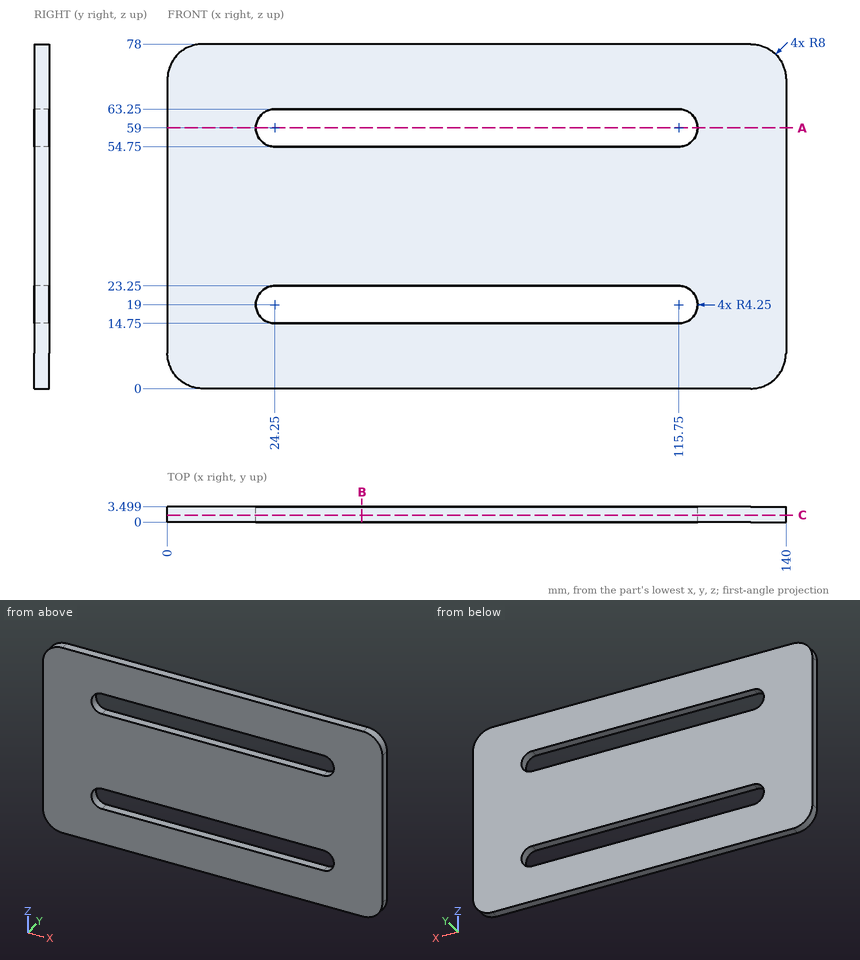
Geometry check sheet. Reference: drawing and pictorial views, mm from the part's lowest x, y, z. Round coordinates to 2 decimals unless told otherwise and drop trailing zeros. Loops run counter-clockwise (first coordinate to the right, second up) from the corner with the lowest first, then second, coordinate; pieces in that order, holes last. Notation, with made-up numbers: M 75.25,60 L 130.25,60 A17 ccw 130.25,79 Z; hole C -30.75,-29 d2. An arc over 180 degrees is marked long. One line per item, written item: value.
(1) Sectioned sample at B-B, the plane x = 44. Record the cut outline in (y, z).
Computed values:
outline: M 0,0 L 3.5,0 L 3.5,14.75 L 0,14.75 Z; M 0,23.25 L 3.5,23.25 L 3.5,54.75 L 0,54.75 Z; M 0,63.25 L 3.5,63.25 L 3.5,78 L 0,78 Z
(2) Thickness scan on line 1 (Z direction, x = 93.5, y = 2.1); line 2 (Z direction, x = 118, y = 1.5) (1 decimal); line 3 (X direction, y = 1, z = 70.5) (1 decimal). Record the ranges inside material, lowest first.
Computed values:
line 1: z = 0 to 14.75, 23.25 to 54.75, 63.25 to 78
line 2: z = 0 to 15.4, 22.6 to 55.4, 62.6 to 78
line 3: x = 0 to 140
(3) Sectioned sample at A-A, the plane z = 59. Record the cut outline in (x, y).
Computed values:
outline: M 0,0 L 20,0 L 20,3.5 L 0,3.5 Z; M 120,0 L 140,0 L 140,3.5 L 120,3.5 Z
(4) Sectioned sample at C-C, the plane y = 1.6. Record the cut outline in (x, z).
Computed values:
outline: M 0,8 A8 ccw 8,0 L 132,0 A8 ccw 140,8 L 140,70 A8 ccw 132,78 L 8,78 A8 ccw 0,70 Z; hole M 24.25,14.75 L 115.75,14.75 A4.25 ccw 115.75,23.25 L 24.25,23.25 A4.25 ccw Z; hole M 24.25,54.75 L 115.75,54.75 A4.25 ccw 115.75,63.25 L 24.25,63.25 A4.25 ccw Z
